Here's how the part is built. I have some questions about the finished solid (model axes, mm). A direction names the side the tool comes from. Give positions to 0.01 mm unless a question says otherwise; leave off trailing zeros. Loops run counter-clockwise (first coordinate to the right, second up) from the corner with the lowest first, then second, coordinate; pieces in that order, holes last.
Q1. For faces 1 (the face through (146, -14, -2)), 2 (the face through (150, -13, -2)), which set-ups out of +Z, -Z, +X, -X, +Y, -Y let a thin tool reach every point of the face, with its end or its side?
Q2. I'm going to push a flat-ended pin straight in: P1, Ø5, axis at x = -69.5, z = -104, coming from the -Y side. Where does the tip first touch, or does it pass through?
Q3. I need wall thicknesses on probe 1 along Z at (x, y) = (111, -23); probe 2 along X at (y, z) = (-11, 72.5); probe 3 along Y at (x, z) = (30.5, -49). Which ranges of each line are inside material? Lowest first, please.
Q4. Suppose I cut it at A-A (y = -12). List the corners of the cut face in (x, z) for me.
Q5. Suppose I cut it at C-C (z = -102). List the corners of the cut face in (x, y) for me.
Q6. Thinking about a two-plate mould opening in Z: for faces 3 (the face through (-2, -13, 138.889)), 4 (the face through (-2, -14, 134.889)), 5 (the face through (-2, -13, -138.889)), which applies, pulls with the +Z half, pulls with the -Z half, needs draft (parallel to the pull), parting line crosses it, or undercut?
Q7. Suppose I cut it at B-B (x = 43.5). List the corners of the cut face in (y, z) for me, and give its area (3 significant figures).
```python
from build123d import *

# Parameters (mm, degrees)
F0_W     = 300
F0_H     = 277.777704
F1_DEPTH = 25
F2_T     = -4
F3_R     = 1.5


with BuildPart() as f1:
    # F0 (on Front) → F1 (new body)
    with BuildSketch(Plane.XZ):
        Rectangle(F0_W, F0_H)
    extrude(amount=F1_DEPTH)

    # F2
    f2_openings = [f1.faces().sort_by_distance(p)[0] for p in [
        (0, -25, 0),
    ]]
    offset(amount=F2_T, openings=f2_openings)

    # F3
    f3_edges = [f1.edges().sort_by_distance(p)[0] for p in [
        (0, 0, -138.888852),
        (150, 0, 0),
        (0, 0, 138.888852),
        (-150, 0, 0),
    ]]
    fillet(f3_edges, radius=F3_R)


solid = f1.part
```
Solutions:
1. face 1: -Y
1. face 2: +Z, -Z, +X, +Y, -Y
2. P1: stops at y = -4
3. probe 1: z = -138.89 to -134.89, 134.89 to 138.89
3. probe 2: x = -150 to -146, 146 to 150
3. probe 3: y = -4 to 0
4. outline: (-150, -138.89) - (150, -138.89) - (150, 138.89) - (-150, 138.89) - close; hole (-146, -134.89) - (146, -134.89) - (146, 134.89) - (-146, 134.89) - close
5. outline: (-150, -25) - (-146, -25) - (-146, -4) - (146, -4) - (146, -25) - (150, -25) - (150, -1.5) arc R1.5 ccw to (148.5, 0) - (-148.5, 0) arc R1.5 ccw to (-150, -1.5) - close
6. face 3: pulls with the +Z half
6. face 4: undercut
6. face 5: pulls with the -Z half
7. outline: (-25, -138.89) - (-1.5, -138.89) arc R1.5 ccw to (0, -137.39) - (0, 137.39) arc R1.5 ccw to (-1.5, 138.89) - (-25, 138.89) - (-25, 134.89) - (-4, 134.89) - (-4, -134.89) - (-25, -134.89) - close
7. area: 1,280 mm2
